from build123d import *

# Parameters (mm, degrees)
SKETCH1_R           = 12.5
BOSS_EXTRUDE2_DEPTH = 12
BOSS_EXTRUDE3_DEPTH = 12
SKETCH3_W           = 8
SKETCH3_H           = 10
CUT_EXTRUDE1_DEPTH  = 10
SKETCH4_R           = 2
CUT_EXTRUDE2_DEPTH  = 14
SKETCH6_R           = 6.125
CUT_EXTRUDE3_DEPTH  = 4
SKETCH7_R           = 2.125
CUT_EXTRUDE4_DEPTH  = 9


with BuildPart() as part:
    # Sketch1 → Boss-Extrude2 (new body)
    with BuildSketch(Plane.XY):
        Circle(SKETCH1_R)
    extrude(amount=BOSS_EXTRUDE2_DEPTH)

    # Sketch2 → Boss-Extrude3 (add)
    with BuildSketch(Plane.XY):
        with BuildLine():
            Line((-24.231440373, 0.295461436), (-11.458506302, -4.995261088))
            ThreePointArc((-11.458506302, -4.995261088), (-12.259311424, 2.441164357), (-8.670952565, 9.003587153))
            Line((-8.670952565, 9.003587153), (-18.87387232, 13.229774891))
            Line((-18.87387232, 13.229774891), (-20.787289482, 8.610377228))
            Line((-20.787289482, 8.610377228), (-24.231440373, 0.295461436))
        make_face()
    extrude(amount=BOSS_EXTRUDE3_DEPTH)

    # Sketch3 → Cut-Extrude1 (cut)
    with BuildSketch(Plane(origin=(-20.787289482, 8.610377228, 0), x_dir=(0, 0, 1), z_dir=(-0.923879533, 0.382683432, 0))):
        with Locations((6, -2)):
            Rectangle(SKETCH3_W, SKETCH3_H)
    extrude(amount=-CUT_EXTRUDE1_DEPTH, mode=Mode.SUBTRACT)

    # Sketch4 → Cut-Extrude2 (cut)
    with BuildSketch(Plane(origin=(1.913417162, 4.619397663, 0), x_dir=(0.923879533, -0.382683432, 0), z_dir=(0.382683432, 0.923879533, 0))):
        with Locations((-16.978219619, -6)):
            Circle(SKETCH4_R)
    extrude(amount=-CUT_EXTRUDE2_DEPTH, mode=Mode.SUBTRACT)

    # Sketch6 → Cut-Extrude3 (cut)
    with BuildSketch(Plane(origin=(0, 0, 0), x_dir=(-1, 0, 0), z_dir=(0, 0, -1))):
        Circle(SKETCH6_R)
    extrude(amount=-CUT_EXTRUDE3_DEPTH, mode=Mode.SUBTRACT)

    # Sketch7 → Cut-Extrude4 (cut, through all)
    with BuildSketch(Plane(origin=(0, 0, 4), x_dir=(-1, 0, 0), z_dir=(0, 0, -1))):
        Circle(SKETCH7_R)
    extrude(amount=-CUT_EXTRUDE4_DEPTH, mode=Mode.SUBTRACT)


solid = part.part
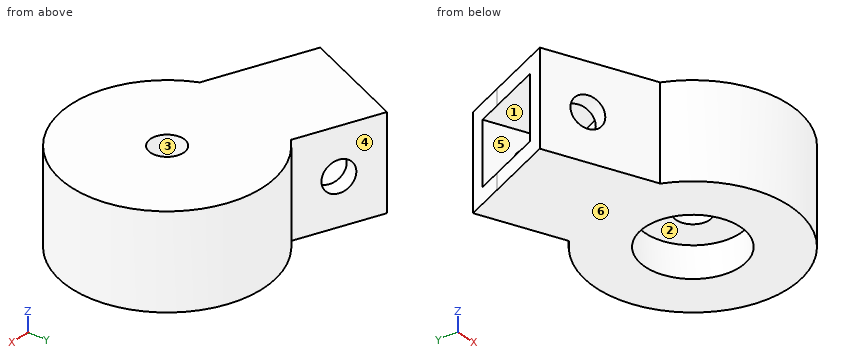
For this review, take the finished solid that the model builds, in its own axes (mm). Face numbers are marked on the shaded views. A direction names the side the tool comes from. Round coordinates to 2 decimals unless told otherwise and drop trailing zeros. Order: outer loops, then holes, each group sorted by start corner. A loop starts at its lowest first (then second) coordinate and runs counter-clockwise, first axis right, second up. Notation, with made-up numbers: M 77,68.5 L 97,68.5 A29 ccw 97,98.5 Z; hole C -6.75,51 d7. An arc over 180 degrees is marked long. Write each question's results on one line, items separated by ' | '. Start each with the question number.
1. Draft analysis for pull direction X (two halves, no side actions). For the marked faces 4, 5 and 6, state which applies: pulls with the +X half, pulls with the -X half, needs draft (parallel to the pull), parting line crosses it, or undercut.
2. Clearance check with flat-ended pins moving along their axes: pin 1 Ø4 at (x, y) = (-14, 6) entering from -Z; pin 2 Ø5 at (y, z) = (-7, 10) entering from -X; pin 3 Ø2 at (y, z) = (6, 10.5) entering from -X. State where each tip first meets the part, or that it passes through.
3. Tool access review of the marked faces 1, 2 and 3: name each direction out of +Z, -Z, +X, -X, +Y, -Y from which nothing blocks a thin tool from reaching the whole face with its end or side.
4. To check wall thickness, follow L1, parallel to Y at x = 0, z = 6 (3 decimals); L2, parallel to Z at x = -17, y = 3.25; L3, parallel to Y at x = 0, z = 1.3 (3 decimals). State the ranges of each line that lie inside material, in increasing order. Write a range as [from, to].
5. Add section A-A (x = 0). State the section outline as (y, z) points (3 decimals).
6. Add section C-C (z = 5). State how many separate pieces and enclosed holes the cut face has, then the cut area to 3 significant figures.
Output values:
1) face 4: undercut | face 5: pulls with the -X half | face 6: needs draft
2) pin 1: z = 0 | pin 2: x = -12.65 | pin 3: x = -22.28
3) face 1: none | face 2: -Z | face 3: +Z, -Z
4) L1: [-12.5, -2.125], [2.125, 12.5] | L2: [0, 2], [10, 12] | L3: [-12.5, -6.125], [6.125, 12.5]
5) outline: M -12.5,0 L -6.125,0 L -6.125,4 L -2.125,4 L -2.125,12 L -12.5,12 Z; M 2.125,4 L 6.125,4 L 6.125,0 L 12.5,0 L 12.5,12 L 2.125,12 Z
6) separate pieces: 3 | enclosed holes: 1 | area: 515 mm^2
